Check sheet for the drawn part. Datum: minimum x, y, z corner. Units: mm. Give positions to 0.01 mm unless a question says otherwise; leave off trailing zeros. Loops run counter-clockwise (first coordinate to the right, second up) from the corner with the lowest first, then second, coordinate; pieces in that order, holes last. Notation, with made-up numbers: (0, -35) - (30, -35) arc R22 ccw to (30, -24) - close; hole circle Ø4 at (24, -17.75). An arc over 180 degrees is marked (long way). Use a Markdown table: item, result. Add a question column.
1. Cross-section at C-C on y = 13.75. Enter the section's corners in (x, z), and give its area (3 significant figures).
2. Cross-section at B-B on z = 2.4. Count the separate pieces of the cut face and the enclosed holes in it, and give its area (3 significant figures).
3. Material ranges on L1, parallel to Y at x = 10, z = 2.15; L2, parallel to X at y = 13.5, z = 2.3; L3, parallel to X at y = 13.25, z = 1.4, recorded low to high.
4. Depth check by flat-ended pin: P1, Ø1.5, axis at y = 12, z = 1.5, coming from the +X side; P2, Ø7, axis at x = 123, y = 10, coming from the +Z side; P3, Ø2, axis at y = 8, z = 2, coming from the -X side; P4, Ø1.5, axis at y = 5, z = 3.5, coming from the -X side. Enter the tip coordinate at first touch or a pass-through.
5. Cross-section at A-A on y = 5.75. Enter the section's corners in (x, z).
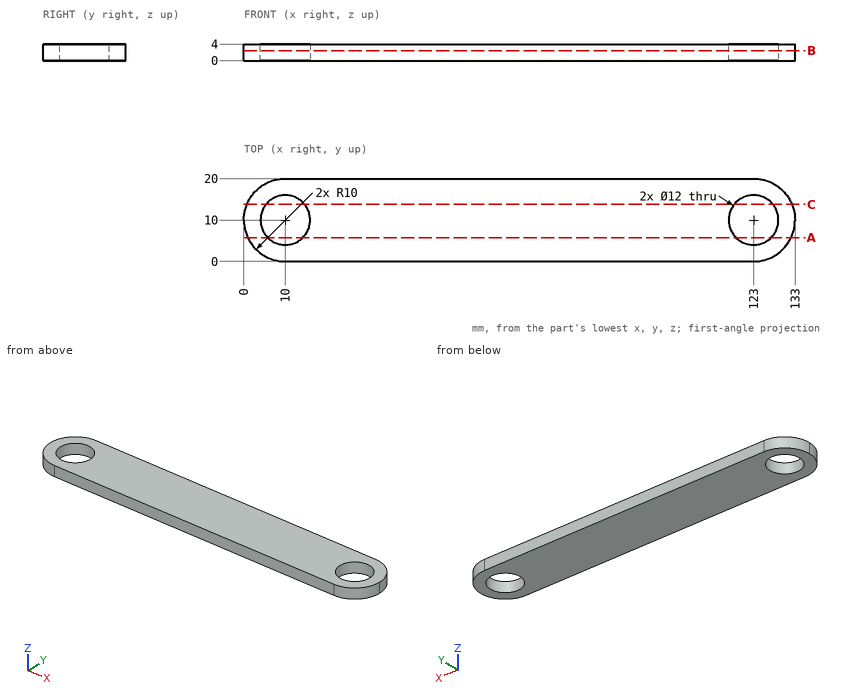
Values found:
| question | item | result |
|---|---|---|
| 1 | outline | (0.73, 0) - (5.32, 0) - (5.32, 4) - (0.73, 4) - close; (14.68, 0) - (118.32, 0) - (118.32, 4) - (14.68, 4) - close; (127.68, 0) - (132.27, 0) - (132.27, 4) - (127.68, 4) - close |
| 1 | area | 451 mm2 |
| 2 | separate pieces | 1 |
| 2 | enclosed holes | 2 |
| 2 | area | 2,350 mm2 |
| 3 | L1 | y = 0 to 4, 16 to 20 |
| 3 | L2 | x = 0.63 to 5.13, 14.87 to 118.13, 127.87 to 132.37 |
| 3 | L3 | x = 0.54 to 4.96, 15.04 to 117.96, 128.04 to 132.46 |
| 4 | P1 | stops at x = 132.92 |
| 4 | P2 | passes through |
| 4 | P3 | stops at x = 0.05 |
| 4 | P4 | stops at x = 0.95 |
| 5 | outline | (0.95, 0) - (5.76, 0) - (5.76, 4) - (0.95, 4) - close; (14.24, 0) - (118.76, 0) - (118.76, 4) - (14.24, 4) - close; (127.24, 0) - (132.05, 0) - (132.05, 4) - (127.24, 4) - close |
